Answer from the drawing. Dimensions are ordinates in mm from the lowest x, y and z of the part. Give positions to 0.01 mm unless a question says otherwise; leave off trailing zeros. Loops run counter-clockwise (first coordinate to the right, second up) from the corner with the lowest first, then second, coordinate; pieces in that order, holes last.
(1) Find section B-B, the plane y = 4.45. State how many separate pieces and enclosed holes the cut face has, then the cut area to 3 significant figures.
(2) Find section A-A, the plane z = 65. Write down the section's boundary in (x, y), then the cut area to 3 significant figures.
(3) Straight lines are drawn through the part: probe 1 along Z at (x, y) = (78, 1.35); probe 2 along X at (y, z) = (4.6, 12); probe 3 along X at (y, z) = (5.3, 80.5). For each, find the intervals that lie inside material, in ascending order.
(4) This flat-tipped pin is pushed along its axis until it touches: P1, Ø3.5, axis at x = 49.5, z = 49.5, coming from the +Y side. Where does it stop, or does it pass through?
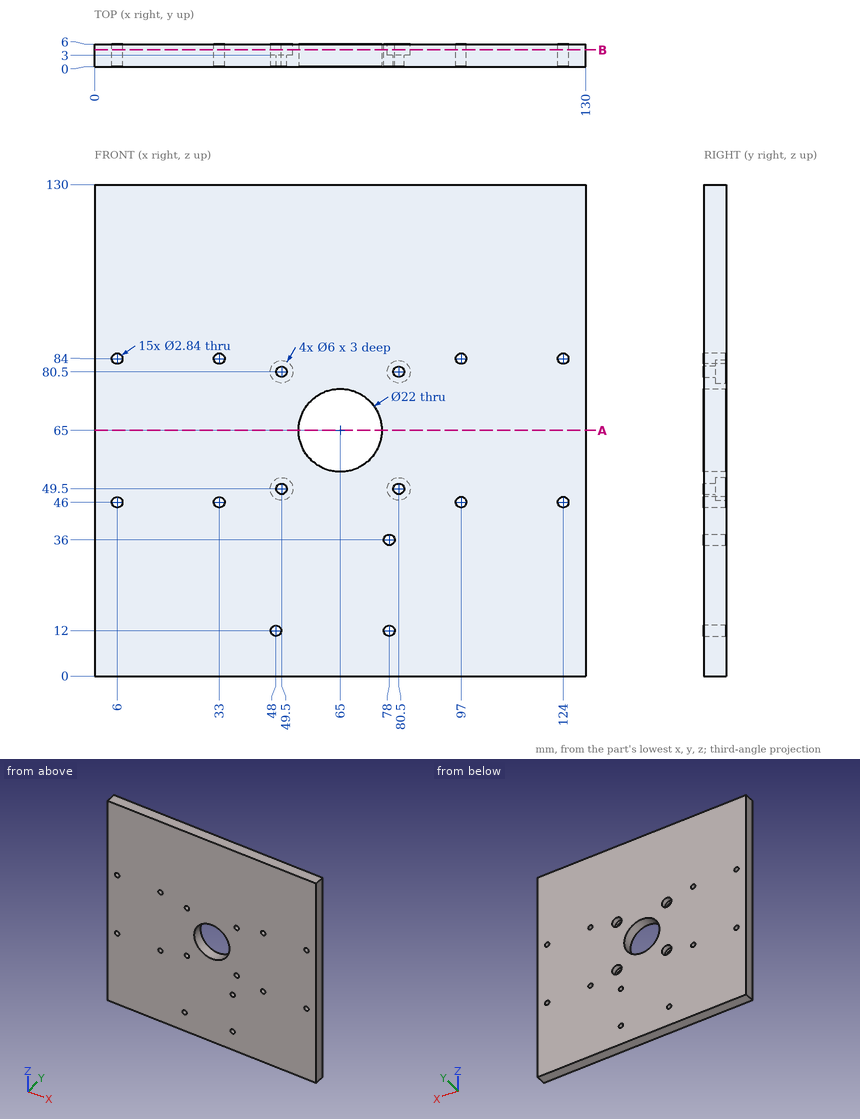
Entries:
1. separate pieces: 1
1. enclosed holes: 16
1. area: 16,300 mm2
2. outline: (0, 0) - (54, 0) - (54, 6) - (0, 6) - close; (76, 0) - (130, 0) - (130, 6) - (76, 6) - close
2. area: 648 mm2
3. probe 1: z = 0 to 10.58, 13.42 to 34.58, 37.42 to 130
3. probe 2: x = 0 to 46.58, 49.42 to 76.58, 79.42 to 130
3. probe 3: x = 0 to 46.5, 52.5 to 77.5, 83.5 to 130
4. P1: stops at y = 3
